The model under review builds one solid part; all positions refer to its coordinate system, in mm. Coordinates: 2 decimals unless noted, no trailing zeros. Write each loop counter-clockwise with the first axis right and the second up, starting at its lowest first coordinate (ties: lowest second). Pieces come first, ordered by that corner, then holes.
```python
from build123d import *

# Parameters (mm, degrees)
SKETCH1_W             = 3.81
SKETCH1_H             = 3.4
BOSS_EXTRUDE1_DEPTH   = 2.5
CUT_EXTRUDE1_DEPTH    = 2.5
CUT_EXTRUDE2_DEPTH    = 2.5
CUT_EXTRUDE3_DEPTH    = 2.5
SKETCH5_W             = 2.4
SKETCH5_H             = 0.1
CUT_EXTRUDE4_DEPTH    = 4.81
CUT_EXTRUDE5_DEPTH    = 2.5
SKETCH7_W             = 0.4
SKETCH7_H             = 0.4
BOSS_EXTRUDE2_DEPTH   = 2.45
SKETCH8_W             = 0.4
SKETCH8_H             = 0.4
BOSS_EXTRUDE3_DEPTH   = 2.45
SKETCH9_W             = 0.4
SKETCH9_H             = 0.4
BOSS_EXTRUDE4_DEPTH   = 2.45
SKETCH10_W            = 0.4
SKETCH10_H            = 0.4
BOSS_EXTRUDE5_DEPTH   = 2.45
SKETCH11_W            = 0.4
SKETCH11_H            = 0.4
BOSS_EXTRUDE6_DEPTH   = 2.45
SKETCH12_W            = 0.4
SKETCH12_H            = 0.4
BOSS_EXTRUDE7_DEPTH   = 2.45
SKETCH13_W            = 0.4
SKETCH13_H            = 0.4
BOSS_EXTRUDE8_DEPTH   = 3
SKETCH14_W            = 0.4
SKETCH14_H            = 0.4
BOSS_EXTRUDE9_DEPTH   = 3
SKETCH15_W            = 0.4
SKETCH15_H            = 0.4
BOSS_EXTRUDE10_DEPTH  = 3
SKETCH16_W            = 0.4
SKETCH16_H            = 0.4
BOSS_EXTRUDE11_DEPTH  = 3
SKETCH17_W            = 0.4
SKETCH17_H            = 0.4
BOSS_EXTRUDE12_DEPTH  = 3
SKETCH18_W            = 0.4
SKETCH18_H            = 0.4
BOSS_EXTRUDE13_DEPTH  = 3
CHAMFER1_SIZE         = 0.15
CHAMFER1_SIZE2        = 0.26
CHAMFER1_PART_2_SIZE  = 0.15
CHAMFER1_PART_2_SIZE2 = 0.26
CHAMFER2_SIZE         = 0.26
CHAMFER2_SIZE2        = 0.15
CHAMFER2_PART_2_SIZE  = 0.26
CHAMFER2_PART_2_SIZE2 = 0.15


with BuildPart() as part:
    # Sketch1 → Boss-Extrude1 (new body)
    with BuildSketch(Plane(origin=(0, 2.5, 0), x_dir=(1, 0, 0), z_dir=(0, 1, 0))):
        with Locations((1.27, 0)):
            Rectangle(SKETCH1_W, SKETCH1_H)
    extrude(amount=-BOSS_EXTRUDE1_DEPTH)

    # Sketch2 → Cut-Extrude1 (cut)
    with BuildSketch(Plane.XZ):
        Polygon((0.785, 1.7), (0.485, 1.7), (0.635, 1.44), align=None)
    extrude(amount=-CUT_EXTRUDE1_DEPTH, mode=Mode.SUBTRACT)

    # Sketch3 → Cut-Extrude2 (cut)
    with BuildSketch(Plane.XZ):
        Polygon((1.755, -1.7), (2.055, -1.7), (1.905, -1.44), align=None)
    extrude(amount=-CUT_EXTRUDE2_DEPTH, mode=Mode.SUBTRACT)

    # Sketch4 → Cut-Extrude3 (cut)
    with BuildSketch(Plane.XZ):
        Polygon((0.485, -1.7), (0.785, -1.7), (0.635, -1.44), align=None)
    extrude(amount=-CUT_EXTRUDE3_DEPTH, mode=Mode.SUBTRACT)

    # Sketch5 → Cut-Extrude4 (cut, through all)
    with BuildSketch(Plane(origin=(3.175, 0, 0), x_dir=(0, 0, -1), z_dir=(1, 0, 0))):
        with Locations((0, 0.05)):
            Rectangle(SKETCH5_W, SKETCH5_H)
    extrude(amount=-CUT_EXTRUDE4_DEPTH, mode=Mode.SUBTRACT)

    # Sketch6 → Cut-Extrude5 (cut)
    with BuildSketch(Plane.XZ):
        Polygon((2.055, 1.7), (1.755, 1.7), (1.905, 1.44), align=None)
    extrude(amount=-CUT_EXTRUDE5_DEPTH, mode=Mode.SUBTRACT)

    # Sketch7 → Boss-Extrude2 (add)
    with BuildSketch(Plane.XZ.offset(-0.1)):
        with Locations((2.54, 0.635)):
            Rectangle(SKETCH7_W, SKETCH7_H)
    extrude(amount=BOSS_EXTRUDE2_DEPTH)

    # Sketch8 → Boss-Extrude3 (add)
    with BuildSketch(Plane.XZ.offset(-0.1)):
        with Locations((2.54, -0.635)):
            Rectangle(SKETCH8_W, SKETCH8_H)
    extrude(amount=BOSS_EXTRUDE3_DEPTH)

    # Sketch9 → Boss-Extrude4 (add)
    with BuildSketch(Plane.XZ.offset(-0.1)):
        with Locations((1.27, 0.635)):
            Rectangle(SKETCH9_W, SKETCH9_H)
    extrude(amount=BOSS_EXTRUDE4_DEPTH)

    # Sketch10 → Boss-Extrude5 (add)
    with BuildSketch(Plane.XZ.offset(-0.1)):
        with Locations((1.27, -0.635)):
            Rectangle(SKETCH10_W, SKETCH10_H)
    extrude(amount=BOSS_EXTRUDE5_DEPTH)

    # Sketch11 → Boss-Extrude6 (add)
    with BuildSketch(Plane.XZ.offset(-0.1)):
        with Locations((0, 0.635)):
            Rectangle(SKETCH11_W, SKETCH11_H)
    extrude(amount=BOSS_EXTRUDE6_DEPTH)

    # Sketch12 → Boss-Extrude7 (add)
    with BuildSketch(Plane.XZ.offset(-0.1)):
        with Locations((0, -0.635)):
            Rectangle(SKETCH12_W, SKETCH12_H)
    extrude(amount=BOSS_EXTRUDE7_DEPTH)

    # Sketch13 → Boss-Extrude8 (add)
    with BuildSketch(Plane(origin=(0, 2.5, 0), x_dir=(-1, 0, 0), z_dir=(0, 1, 0))):
        with Locations((-2.54, 0.635)):
            Rectangle(SKETCH13_W, SKETCH13_H)
    extrude(amount=BOSS_EXTRUDE8_DEPTH)

    # Sketch14 → Boss-Extrude9 (add)
    with BuildSketch(Plane(origin=(0, 2.5, 0), x_dir=(-1, 0, 0), z_dir=(0, 1, 0))):
        with Locations((-2.54, -0.635)):
            Rectangle(SKETCH14_W, SKETCH14_H)
    extrude(amount=BOSS_EXTRUDE9_DEPTH)

    # Sketch15 → Boss-Extrude10 (add)
    with BuildSketch(Plane(origin=(0, 2.5, 0), x_dir=(-1, 0, 0), z_dir=(0, 1, 0))):
        with Locations((-1.27, 0.635)):
            Rectangle(SKETCH15_W, SKETCH15_H)
    extrude(amount=BOSS_EXTRUDE10_DEPTH)

    # Sketch16 → Boss-Extrude11 (add)
    with BuildSketch(Plane(origin=(0, 2.5, 0), x_dir=(-1, 0, 0), z_dir=(0, 1, 0))):
        with Locations((-1.27, -0.635)):
            Rectangle(SKETCH16_W, SKETCH16_H)
    extrude(amount=BOSS_EXTRUDE11_DEPTH)

    # Sketch17 → Boss-Extrude12 (add)
    with BuildSketch(Plane(origin=(0, 2.5, 0), x_dir=(-1, 0, 0), z_dir=(0, 1, 0))):
        with Locations((0, 0.635)):
            Rectangle(SKETCH17_W, SKETCH17_H)
    extrude(amount=BOSS_EXTRUDE12_DEPTH)

    # Sketch18 → Boss-Extrude13 (add)
    with BuildSketch(Plane(origin=(0, 2.5, 0), x_dir=(-1, 0, 0), z_dir=(0, 1, 0))):
        with Locations((0, -0.635)):
            Rectangle(SKETCH18_W, SKETCH18_H)
    extrude(amount=BOSS_EXTRUDE13_DEPTH)

    # Chamfer1
    chamfer1_edges = [part.edges().sort_by_distance(p)[0] for p in [
        (-0.635, 1.25, 1.7),
    ]]
    chamfer1_side = [part.faces().sort_by_distance(p)[0] for p in [
        (-0.075, 1.25, 1.7),
    ]]
    chamfer(chamfer1_edges, length=CHAMFER1_SIZE, length2=CHAMFER1_SIZE2, reference=chamfer1_side[0])

    # Chamfer1 part 2
    chamfer1_part_2_edges = [part.edges().sort_by_distance(p)[0] for p in [
        (3.175, 1.25, -1.7),
    ]]
    chamfer1_part_2_side = [part.faces().sort_by_distance(p)[0] for p in [
        (2.615, 1.25, -1.7),
    ]]
    chamfer(chamfer1_part_2_edges, length=CHAMFER1_PART_2_SIZE, length2=CHAMFER1_PART_2_SIZE2, reference=chamfer1_part_2_side[0])

    # Chamfer2
    chamfer2_edges = [part.edges().sort_by_distance(p)[0] for p in [
        (-0.635, 1.25, -1.7),
    ]]
    chamfer2_side = [part.faces().sort_by_distance(p)[0] for p in [
        (-0.635, 1.287844941, -0.134099869),
    ]]
    chamfer(chamfer2_edges, length=CHAMFER2_SIZE, length2=CHAMFER2_SIZE2, reference=chamfer2_side[0])

    # Chamfer2 part 2
    chamfer2_part_2_edges = [part.edges().sort_by_distance(p)[0] for p in [
        (3.175, 1.25, 1.7),
    ]]
    chamfer2_part_2_side = [part.faces().sort_by_distance(p)[0] for p in [
        (3.175, 1.287844941, 0.134099869),
    ]]
    chamfer(chamfer2_part_2_edges, length=CHAMFER2_PART_2_SIZE, length2=CHAMFER2_PART_2_SIZE2, reference=chamfer2_part_2_side[0])


solid = part.part
```
Item 1: Take a section at A-A, the plane y = 3.25. Write out the cut boundary in (x, z) (3 decimals), plus the area to 3 significant figures.
Solved:
outline: (-0.2, -0.835) - (0.2, -0.835) - (0.2, -0.435) - (-0.2, -0.435) - close; (-0.2, 0.435) - (0.2, 0.435) - (0.2, 0.835) - (-0.2, 0.835) - close; (1.07, -0.835) - (1.47, -0.835) - (1.47, -0.435) - (1.07, -0.435) - close; (1.07, 0.435) - (1.47, 0.435) - (1.47, 0.835) - (1.07, 0.835) - close; (2.34, -0.835) - (2.74, -0.835) - (2.74, -0.435) - (2.34, -0.435) - close; (2.34, 0.435) - (2.74, 0.435) - (2.74, 0.835) - (2.34, 0.835) - close
area: 0.960 mm2
Item 2: To check wall thickness, follow line 1 along X through (y, z) = (3.5, 0.7); line 2 along Z through (x, y) = (0, 4) (3 decimals); line 3 along Y through (x, z) = (1.1, -0.25). State the ranges of each line that lie inside material, in increasing order.
Solved:
line 1: x = -0.2 to 0.2, 1.07 to 1.47, 2.34 to 2.74
line 2: z = -0.835 to -0.435, 0.435 to 0.835
line 3: y = 0.1 to 2.5
Item 3: Take a section at B-B, the plane z = 0.7. Write out the cut boundary in (x, y) (3 decimals), plus the area to 3 significant figures.
Solved:
outline: (-0.635, 0.1) - (-0.2, 0.1) - (-0.2, -2.35) - (0.2, -2.35) - (0.2, 0.1) - (1.07, 0.1) - (1.07, -2.35) - (1.47, -2.35) - (1.47, 0.1) - (2.34, 0.1) - (2.34, -2.35) - (2.74, -2.35) - (2.74, 0.1) - (3.175, 0.1) - (3.175, 2.5) - (2.74, 2.5) - (2.74, 5.5) - (2.34, 5.5) - (2.34, 2.5) - (1.47, 2.5) - (1.47, 5.5) - (1.07, 5.5) - (1.07, 2.5) - (0.2, 2.5) - (0.2, 5.5) - (-0.2, 5.5) - (-0.2, 2.5) - (-0.635, 2.5) - close
area: 15.7 mm2
Item 4: Mouldability with a two-part tool opening along Z and no side actions: class faces 1 (the face through (1, 0.1, 0)), 2 (the face through (1, 1, 1.7)), 3 (the face through (0, 1, -1.7)) as pulls with the +Z half, pulls with the -Z half, needs draft (parallel to the pull), parting line crosses it, or undercut.
Solved:
face 1: undercut
face 2: pulls with the +Z half
face 3: pulls with the -Z half
Item 5: Take a section at C-C, the plane x = -0.4. Write out the cut boundary in (y, z), plus the area to 3 significant figures.
Solved:
outline: (0, -1.7) - (2.5, -1.7) - (2.5, 1.7) - (0, 1.7) - (0, 1.2) - (0.1, 1.2) - (0.1, -1.2) - (0, -1.2) - close
area: 8.26 mm2
Item 6: Take a section at D-D, the plane y = 0.5. Write out the cut boundary in (x, z) (3 decimals), plus the area to 3 significant figures.
Solved:
outline: (-0.635, -1.44) - (-0.485, -1.7) - (0.485, -1.7) - (0.635, -1.44) - (0.785, -1.7) - (1.755, -1.7) - (1.905, -1.44) - (2.055, -1.7) - (3.025, -1.7) - (3.175, -1.44) - (3.175, 1.44) - (3.025, 1.7) - (2.055, 1.7) - (1.905, 1.44) - (1.755, 1.7) - (0.785, 1.7) - (0.635, 1.44) - (0.485, 1.7) - (-0.485, 1.7) - (-0.635, 1.44) - close
area: 12.7 mm2
